The drawing under review shows one solid part. Ordinate dimensions are in mm from its lowest x, y, z. A direction names the side the tool comes from. Coordinates: 2 decimals unless noted, no trailing zeros. Loops run counter-clockwise (first coordinate to the right, second up) from the corner with the lowest first, then second, coordinate; pieces in that order, holes last. Notation, with made-up numbers: M 40,5 L 91,5 A10 cw 91,9 Z; hole C -36,60 d8. An arc over 180 degrees is marked long. Put each result on its own line as item: value.
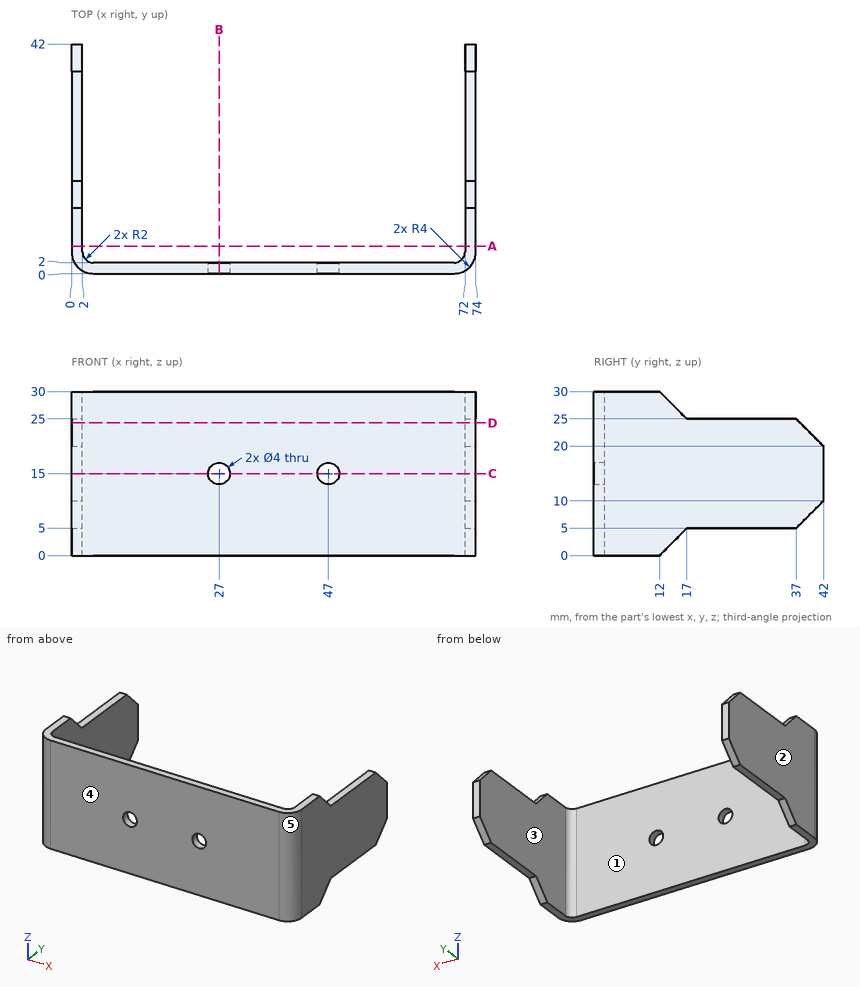
(1) Add section A-A (y = 5). Write out the cut boundary in (x, z).
Determined:
outline: M 0,0 L 2,0 L 2,30 L 0,30 Z; M 72,0 L 74,0 L 74,30 L 72,30 Z
(2) Tool access review of the marked faces 1 and 2: name each direction out of +Z, -Z, +X, -X, +Y, -Y from which nothing blocks a thin tool from reaching the whole face with its end or side.
Determined:
face 1: +Z, -Z, +Y
face 2: +Z, -Z, -X, +Y, -Y
(3) For pin 1 (4.5 mm diameter, centred on x = 27, z = 15, fed in from +Y); pin 2 (0.6 mm diameter, centred on x = 72.5, y = 28, fed in from +Z); pin 3 (1 mm diameter, centred on x = 73, y = 24, fed in from -Z); pin 4 (12 mm diameter, centred on x = 61.5, y = 16.5, fed in from +Z), all flat-tipped, find the tip position at first contact; note any pin that passes through.
Determined:
pin 1: stops at y = 2
pin 2: stops at z = 25
pin 3: stops at z = 5
pin 4: passes through
(4) Draft analysis for pull direction X (two halves, no side actions). For the marked faces 3, 4 and 5, state which applies: +X half, -X half, draft (parallel to the pull), parting line (faces both ways), or undercut.
Determined:
face 3: undercut
face 4: draft
face 5: +X half
(5) Add section D-D (z = 24.25). Write out the cut boundary in (x, y), plus the area to 3 significant figures.
Determined:
outline: M 0,4 A4 ccw 4,0 L 70,0 A4 ccw 74,4 L 74,37.75 L 72,37.75 L 72,4 A2 cw 70,2 L 4,2 A2 cw 2,4 L 2,37.75 L 0,37.75 Z
area: 286 mm^2
(6) Add section C-C (z = 15). Write out the cut boundary in (x, y), plus the area to 3 significant figures.
Determined:
outline: M 0,4 A4 ccw 4,0 L 25,0 L 25,2 L 4,2 A2 cw 2,4 L 2,42 L 0,42 Z; M 29,0 L 45,0 L 45,2 L 29,2 Z; M 49,0 L 70,0 A4 ccw 74,4 L 74,42 L 72,42 L 72,4 A2 cw 70,2 L 49,2 Z
area: 287 mm^2
(7) Add section B-B (x = 27). Write out the cut boundary in (y, z), plus the area to 3 significant figures.
Determined:
outline: M 0,0 L 2,0 L 2,13 L 0,13 Z; M 0,17 L 2,17 L 2,30 L 0,30 Z
area: 52.0 mm^2
(8) Wall thickness on line 1 along X through (y, z) = (11.5, 18.5); line 2 along X through (y, z) = (1.4, 15); line 3 along X through (y, z) = (0.85, 15): over which ranges is each line inside the solid? List them lowest first. Write a range as [from, to].
Determined:
line 1: x = [0, 2], [72, 74]
line 2: x = [0.96, 25], [29, 45], [49, 73.04]
line 3: x = [1.53, 25], [29, 45], [49, 72.47]
